```python
from build123d import *

# Parameters (mm, degrees)
PAD_DEPTH       = 20
SKETCH001_R     = 2.25
POCKET_DEPTH    = 15.001
SKETCH002_R     = 5
POCKET001_DEPTH = 3


with BuildPart() as part:
    # Sketch → Pad (new body)
    with BuildSketch(Plane.XY):
        with BuildLine():
            ThreePointArc((-6.05, 0), (0, -6.05), (6.05, 0))
            Line((6.05, 0), (17.5, 0))
            Line((17.5, 0), (17.5, -15))
            Line((17.5, -15), (-17.5, -15))
            Line((-17.5, -15), (-17.5, 0))
            Line((-17.5, 0), (-6.05, 0))
        make_face()
    extrude(amount=PAD_DEPTH)

    # Sketch001 → Pocket (cut, through all)
    with BuildSketch(Plane.XZ.offset(15)):
        with Locations((-11, 10)):
            Circle(SKETCH001_R)
        with Locations((11, 10)):
            Circle(SKETCH001_R)
    extrude(amount=-POCKET_DEPTH, mode=Mode.SUBTRACT)

    # Sketch002 → Pocket001 (cut)
    with BuildSketch(Plane.XZ.offset(15)):
        with Locations((-11.052364, 10)):
            Circle(SKETCH002_R)
        with Locations((10.947636, 10)):
            Circle(SKETCH002_R)
    extrude(amount=-POCKET001_DEPTH, mode=Mode.SUBTRACT)


solid = part.part
```
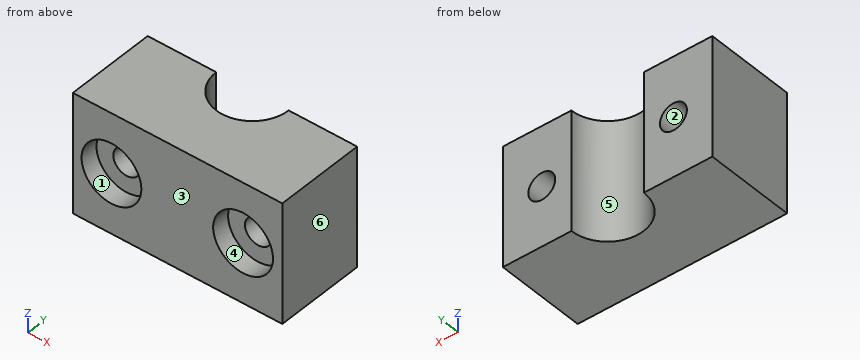
Model file for the job. Use its own axes, mm. Face numbers are marked on the shaded views. A direction names the side the tool comes from. Coordinates: 2 decimals unless noted, no trailing zeros. Write each loop counter-clockwise with the first axis right and the second up, starting at its lowest first coordinate (ties: lowest second). Pieces come first, ordered by that corner, then holes. Notation, with made-up numbers: (40.25, 62) - (96.25, 62) arc R25 cw to (96.25, 80) - close; hole circle Ø4 at (84, 72). An arc over 180 degrees is marked (long way). One line per question, with ' | ' between items. Start each with the question number.
Q1. Cut at D-D, the plane y = -13.5. List the corners of the cut face in (x, z), then the cut area to 3 significant figures.
Q2. Pin check, flat tips, straight feed: pin 1 (6 mm diameter, centred on x = -11.05, z = 10, fed in from -Y); pin 2 (2.5 mm diameter, centred on x = -11, z = 10, fed in from +Y); pin 3 (4 mm diameter, centred on x = -3.5, z = 7, fed in from +Y). Stop position of each tip, or through.
Q3. 3-axis set-ups, long thin cutter, end or side, ignore diameter. For the marked faces 1 and 2: which of +Z, -Z, +X, -X, +Y, -Y reach the whole face in a straight line?
Q4. Cut at C-C, the plane x = 12. List the corners of the cut face in (y, z).
Q5. Pull direction X, two halves, no side cores. Call the marked faces 3, 4, 5 and 6: pulls with the +X half, pulls with the -X half, needs draft (parallel to the pull), parting line crosses it, or undercut.
Q6. Cut at B-B, the plane z = 10. List the corners of the cut face in (x, y), then the cut area to 3 significant figures.
Q7. Cut at A-A, the plane y = -5.25. List the corners of the cut face in (x, z).
Q8. Drill centre lines: line 1 (X direction, y = -11.75, z = 9.5); line 2 (Y direction, x = 8.5, z = 11.75); line 3 (X direction, y = -5.25, z = 12.5). Where is each one in solid material? Low to high. Write a range as [from, to].
Answer below:
1) outline: (-17.5, 0) - (17.5, 0) - (17.5, 20) - (-17.5, 20) - close; hole circle Ø10 at (-11.05, 10); hole circle Ø10 at (10.95, 10) | area: 543 mm^2
2) pin 1: y = -12 | pin 2: through | pin 3: y = -2.52
3) face 1: -Y | face 2: +Y, -Y
4) outline: (-15, 0) - (0, 0) - (0, 7.98) - (-12, 7.98) - (-12, 5.11) - (-15, 5.11) - close; (-15, 14.89) - (-12, 14.89) - (-12, 12.02) - (0, 12.02) - (0, 20) - (-15, 20) - close
5) face 3: needs draft | face 4: undercut | face 5: undercut | face 6: pulls with the +X half
6) outline: (-17.5, -15) - (-16.05, -15) - (-16.05, -12) - (-13.25, -12) - (-13.25, 0) - (-17.5, 0) - close; (-8.75, -12) - (-6.05, -12) - (-6.05, -15) - (5.95, -15) - (5.95, -12) - (8.75, -12) - (8.75, 0) - (6.05, 0) arc R6.05 cw to (-6.05, 0) - (-8.75, 0) - close; (13.25, -12) - (15.95, -12) - (15.95, -15) - (17.5, -15) - (17.5, 0) - (13.25, 0) - close | area: 300 mm^2
7) outline: (-17.5, 0) - (-3.01, 0) - (-3.01, 20) - (-17.5, 20) - close; (3.01, 0) - (17.5, 0) - (17.5, 20) - (3.01, 20) - close; hole circle Ø4.5 at (-11, 10); hole circle Ø4.5 at (11, 10)
8) line 1: [-17.5, -13.19], [-8.81, 8.81], [13.19, 17.5] | line 2: [-12, 0] | line 3: [-17.5, -3.01], [3.01, 17.5]
